Autodesk Inventor part; units mm, degrees
ref_plane "YZ Plane" through (0, 0, 0) normal (1, 0, 0) x (0, 1, 0)
ref_plane "XZ Plane" through (0, 0, 0) normal (0, 1, 0) x (-1, 0, 0)
ref_plane "XY Plane" through (0, 0, 0) normal (0, 0, 1) x (1, 0, 0)
ref_plane "Work Plane1" through (223.0039, -4.7048, -1.4) normal (0, 0, 1) x (1, 0, 0)
sketch "Sketch1" plane through (223.0039, -4.7048, -1.4) normal (0, 0, 1) x (1, 0, 0)
  arc A0 (6.5712, 0.3844) -> (6.5712, 1.6156) centre (0, 1) ccw
  line L0 (-6.5712, 0.3844) -> (-4.25, -24.3945)
  arc A1 (-4.25, -24.3945) -> (4.25, -24.3945) centre (0, -23.9964) ccw
  line L1 (4.25, -24.3945) -> (6.5712, 0.3844)
  line L2 (0, 1) -> (-6.6, 1) construction
  line L3 (-6.5712, 1.6156) -> (-4.25, 26.3945)
  arc A2 (4.25, 26.3945) -> (-4.25, 26.3945) centre (0, 25.9964) ccw
  line L4 (4.25, 26.3945) -> (6.5712, 1.6156)
  arc A3 (-6.5712, 0.3844) -> (6.5712, 0.3844) centre (0, 1) ccw construction
  arc A4 (-6.5712, 1.6156) -> (-6.5712, 0.3844) centre (0, 1) ccw
  arc A5 (6.5712, 1.6156) -> (-6.5712, 1.6156) centre (0, 1) ccw construction
  circle A6 centre (0, 1) radius 2.5 construction
  point P0 (-223.0039, 4.7048)
  point P1 (0, -28.265)
  dimension "d0" = 13.2
  dimension "d1" = 8.5
  dimension "d2" = 30
extrude "Extrusion1" add sketch "Sketch1" along normal blind 2.6
sketch "Sketch2" plane through (223.0039, -4.7048, -1.4) normal (0, 0, -1) x (-1, 0, 0)
  arc A0 (6.5712, 1.6156) -> (-6.5712, 1.6156) centre (0, 1) ccw
  arc A1 (-6.5712, 1.6156) -> (-6.5712, 0.3844) centre (0, 1) ccw
  arc A2 (-6.5712, 0.3844) -> (6.5712, 0.3844) centre (0, 1) ccw
  arc A3 (6.5712, 0.3844) -> (6.5712, 1.6156) centre (0, 1) ccw
  line L0 (-4.875, -9) -> (4.875, -9)
  line L1 (4.875, -9) -> (4.875, 11)
  line L2 (4.875, 11) -> (-4.875, 11)
  line L3 (-4.875, 11) -> (-4.875, -9)
  line L4 (-4.875, -9) -> (4.875, 11) construction
  point P0 (4.875, 5.4491)
  point P1 (4.875, -3.4491)
  point P2 (-4.875, -3.4491)
  point P3 (-4.875, 5.4491)
  dimension "d5" = 9.75
  dimension "d6" = 20
extrude "Extrusion2" add sketch "Sketch2" along normal blind 1
ref_plane "Work Plane2" through (223.0039, -4.7048, -0.1) normal (0, 0, 1) x (1, 0, 0)
mirror "Mirror1" about plane through (223.0039, -4.7048, -0.1) normal (0, 0, 1) of "Extrusion2"
sketch "Sketch3" plane through (218.1289, 6.2952, 2.2) normal (0, 0, 1) x (1, 0, 0)
  arc A0 (0, -5.5509) -> (0, -14.4491) centre (4.875, -10) ccw
  arc A1 (0, -5.5509) -> (0, -14.4491) centre (4.875, -10) ccw
  circle A2 centre (4.875, -10) radius 3.75
  point P0 (-218.1289, -6.2952)
  point P1 (0, -16.5009)
  point P2 (9.75, -16.5009)
  point P3 (9.75, -14.4491)
  point P4 (9.75, -14.4491)
  point P5 (9.75, 1.9491)
  point P6 (9.75, -5.5509)
  dimension "d9" = 7.5
extrude "Extrusion3" add sketch "Sketch3" along normal blind 3.5
properties part number "Servo Horn"
Design review of the part built by this model. Coordinates are the model's own, in mm. A direction names the side the tool comes from. Give positions to 0.01 mm unless a question says otherwise; leave off trailing zeros. Order: outer loops, then holes, each group sorted by start corner. A loop starts at its lowest first (then second) coordinate and runs counter-clockwise, first axis right, second up. Notation, with made-up numbers: (75, 17.25) -> (104, 17.25) arc R10 ccw to (104, 36.25) -> close; hole circle Ø6 at (82.25, -29). An arc over 180 degrees is marked (long way). Write each question's results on one line, items separated by ' | '. Start each with the question number.
Q1. For pin 1 (1 mm diameter, centred on y = 12, z = 1.5, fed in from +X); pin 2 (3 mm diameter, centred on x = 225, y = 17, fed in from +Z); pin 3 (0.8 mm diameter, centred on x = 222, z = 2, fed in from -Y); pin 4 (2 mm diameter, centred on y = 14, z = 3.5, fed in from +X), all flat-tipped, find the tip position at first contact; note any pin that passes through.
Q2. Mouldability with a two-part tool opening along Z and no side actions: class faces 6 (the flat face through (223, -13.705, -2)), 7 (the flat face through (223, -4, 5.7)), 8 (the flat face through (223, -4, -2.4)) as +Z half, -Z half, draft (parallel to the pull), parting line (faces both ways), or undercut.
Q3. Wall thickness on L1, parallel to Z at x = 226.75, y = -4.5; L2, parallel to Z at x = 220, y = -25.5; L3, parallel to Y at x = 223.25, z = 3: over which ranges is each line inside the solid? List them lowest first. Write a range as from..to.
Q4. Add section D-D on z = 3.75. Give the boundary of the cut face in (x, y), and give its area (3 significant figures).
Q5. Add section B-B on x = 224.75. Give the boundary of the cut face in (y, z), and give its area (3 significant figures).
Q6. Machinability: for faces 1 (the flat face through (223, 6.295, -2)), 2 (the flat face through (227.879, 3, 2)), 3 (the flat face through (223, 6.295, 2)), 4 (the flat face through (227.879, -11, -2)), 5 (the cylindrical face through (226.47, -2.27, 3.93)), which of the approach directions +Z, -Z, +X, -X, +Y, -Y give a long, thin tool a straight path to every point of the face, cutting with its end or side? Answer none if there is none.
Q7. Add section A-A on z = -0.5. Give the boundary of the cut face in (x, y).
Found:
1) pin 1: stops at x = 228.2 | pin 2: stops at z = 1.2 | pin 3: stops at y = -13.7 | pin 4: passes through
2) face 6: draft | face 7: +Z half | face 8: -Z half
3) L1: z = -2.4..2.2 | L2: z = -1.4..1.2 | L3: y = -7.45..0.04
4) outline: circle Ø7.5 at (223, -3.7) | area: 44.2 mm2
5) outline: (-32.6, -1.4) -> (-13.7, -1.4) -> (-13.7, -2.4) -> (6.3, -2.4) -> (6.3, -1.4) -> (25.19, -1.4) -> (25.19, 1.2) -> (6.3, 1.2) -> (6.3, 2.2) -> (-0.39, 2.2) -> (-0.39, 5.7) -> (-7.02, 5.7) -> (-7.02, 2.2) -> (-13.7, 2.2) -> (-13.7, 1.2) -> (-32.6, 1.2) -> close | area: 213 mm2
6) face 1: -Z, +X, -X, +Y | face 2: +Z, +X, +Y | face 3: +Z, +X, -X, +Y | face 4: -Z, +X, -Y | face 5: +Z
7) outline: (216.43, -4.32) -> (218.75, -29.1) arc R4.27 ccw to (227.25, -29.1) -> (229.58, -4.32) arc R6.6 ccw to (229.58, -3.09) -> (227.25, 21.69) arc R4.27 ccw to (218.75, 21.69) -> (216.43, -3.09) arc R6.6 ccw to start
